Input: part model. Units: mm. Frame: model coordinates. A direction names the side the tool comes from. Coordinates: 2 decimals unless noted, no trailing zeros. Loops run counter-clockwise (first coordinate to the right, second up) from the corner with the lowest first, then second, coordinate; pieces in that order, holes last. Notation, with made-up numbers: (30.5, 40.5) -> (60.5, 40.5) arc R10 cw to (60.5, 50.5) -> close; hole circle Ø5 at (-35, 66). An arc over 180 degrees is marked (long way). Answer as a JSON object with one key per item and string values.
from build123d import *

# Parameters (mm, degrees)
BOSS_EXTRUDE1_DEPTH                 = 31.75
SKETCH3_W                           = 25.4
SKETCH3_H                           = 25.4
CUT_EXTRUDE1_DEPTH                  = 25.4
CUT_EXTRUDE2_DEPTH                  = 30.48
SKETCH5_W                           = 2.54
SKETCH5_H                           = 2.54
BOSS_EXTRUDE2_DEPTH                 = 2.032
SKETCH7_W                           = 2.54
SKETCH7_H                           = 2.54
BOSS_EXTRUDE3_DEPTH                 = 2.032
FILLET1_R                           = 2.54
FILLET2_R                           = 2.54
TAP_DRILL_FOR_6_32_TAP1_D           = 2.7051
TAP_DRILL_FOR_6_32_TAP1_CSINK_D     = 3.9751
TAP_DRILL_FOR_6_32_TAP1_CSINK_ANGLE = 90
TAP_DRILL_FOR_6_32_TAP2_D           = 2.7051
TAP_DRILL_FOR_6_32_TAP2_CSINK_D     = 3.9751
TAP_DRILL_FOR_6_32_TAP2_CSINK_ANGLE = 90


with BuildPart() as part:
    # Sketch1 → Boss-Extrude1 (new, symmetric)
    with BuildSketch(Plane(origin=(0, 0, 0), x_dir=(1, 0, 0), z_dir=(0, 1, 0))):
        with BuildLine():
            Line((-4.43094419, 12.953042159), (-15.24, 12.953042159))
            Line((-15.24, 12.953042159), (-15.24, -16.51))
            Line((-15.24, -16.51), (15.24, -16.51))
            Line((15.24, -16.51), (15.24, 12.953042159))
            Line((15.24, 12.953042159), (4.43094419, 12.953042159))
            ThreePointArc((4.43094419, 12.953042159), (0, 12.82766418), (-4.43094419, 12.953042159))
        make_face()
        with BuildLine():
            Line((-15.24, 14.323960084), (-15.24, 12.953042159))
            Line((-15.24, 12.953042159), (-4.43094419, 12.953042159))
            ThreePointArc((-4.43094419, 12.953042159), (-9.859328847, 13.450401628), (-15.24, 14.323960084))
        make_face()
        with BuildLine():
            ThreePointArc((15.24, 14.323960084), (9.859328847, 13.450401628), (4.43094419, 12.953042159))
            Line((4.43094419, 12.953042159), (15.24, 12.953042159))
            Line((15.24, 12.953042159), (15.24, 14.323960084))
        make_face()
    extrude(amount=BOSS_EXTRUDE1_DEPTH, both=True)

    # Sketch3 → Cut-Extrude1 (cut)
    with BuildSketch(Plane.XY.offset(16.51)):
        with Locations((0, -16.51)):
            Rectangle(SKETCH3_W, SKETCH3_H)
    extrude(amount=-CUT_EXTRUDE1_DEPTH, mode=Mode.SUBTRACT)

    # Sketch4 → Cut-Extrude2 (cut)
    with BuildSketch(Plane(origin=(15.24, 0, 0), x_dir=(0, 0, -1), z_dir=(1, 0, 0))):
        Polygon((-16.51, 31.75), (14.323960084, 31.75), (-16.51, 0), align=None)
    extrude(amount=-CUT_EXTRUDE2_DEPTH, mode=Mode.SUBTRACT)

    # Sketch5 → Boss-Extrude2 (add)
    with BuildSketch(Plane(origin=(15.24, 0, 0), x_dir=(0, 0, -1), z_dir=(1, 0, 0))):
        with Locations((-13.616039916, -25.4)):
            Rectangle(SKETCH5_W, SKETCH5_H)
        with Locations((-13.616039916, -15.24)):
            Rectangle(SKETCH5_W, SKETCH5_H)
    extrude(amount=BOSS_EXTRUDE2_DEPTH)

    # Sketch7 → Boss-Extrude3 (add)
    with BuildSketch(Plane.ZY.offset(15.24)):
        with Locations((13.616039916, -25.4)):
            Rectangle(SKETCH7_W, SKETCH7_H)
        with Locations((13.616039916, -15.24)):
            Rectangle(SKETCH7_W, SKETCH7_H)
    extrude(amount=BOSS_EXTRUDE3_DEPTH)

    # Sketch21 → #1 (0.228) Diameter Hole3 (revolve, cut)
    with BuildSketch(Plane(origin=(0, -3.81, 3.81), x_dir=(0, 0, -1), z_dir=(1, 0, 0))):
        Polygon((0, 0), (0, 35.56), (2.8956, 35.56), (2.8956, 0.12065), (3.01625, 0), align=None)
    revolve(axis=Axis((0, -10.16, 3.81), (0, 1, 0)), mode=Mode.SUBTRACT)

    # Fillet1
    fillet1_edges = [part.edges().sort_by_distance(p)[0] for p in [
        (0, 0, 16.51),
    ]]
    fillet(fillet1_edges, radius=FILLET1_R)

    # Fillet2
    fillet2_edges = [part.edges().sort_by_distance(p)[0] for p in [
        (0, -31.75, 16.51),
    ]]
    fillet(fillet2_edges, radius=FILLET2_R - 0.0001)  # a hair under: the kernel refuses the full size

    # Tap Drill for #6-32 Tap1 (through all)
    with Locations(Plane.XY.offset(-8.89)):
        with Locations((-8.688147052, -16.814161917)):
            CounterSinkHole(TAP_DRILL_FOR_6_32_TAP1_D / 2, TAP_DRILL_FOR_6_32_TAP1_CSINK_D / 2, counter_sink_angle=TAP_DRILL_FOR_6_32_TAP1_CSINK_ANGLE)

    # Tap Drill for #6-32 Tap2 (through all)
    with Locations(Plane.XY.offset(-8.89)):
        with Locations((8.657032922, -16.667582931)):
            CounterSinkHole(TAP_DRILL_FOR_6_32_TAP2_D / 2, TAP_DRILL_FOR_6_32_TAP2_CSINK_D / 2, counter_sink_angle=TAP_DRILL_FOR_6_32_TAP2_CSINK_ANGLE)


solid = part.part
1. Section query C-C (y = 9.5). Return loops of the section in (x, z).
Reply:
{"outline": "(-15.24, -14.32) arc R78.36 cw to (15.24, -14.32) -> (15.24, 7.28) -> (-15.24, 7.28) -> close; hole circle Ø5.79 at (0, 3.81)"}
2. Section query A-A (z = -4.5). Return loops of the section in (x, y).
Reply:
{"outline": "(-15.24, -31.75) -> (15.24, -31.75) -> (15.24, 21.63) -> (-15.24, 21.63) -> close; hole (-12.7, -29.21) -> (12.7, -29.21) -> (12.7, -3.81) -> (-12.7, -3.81) -> close"}
3. Access query for faces 1 (the face through (-16, -15, 14.886)), 2 (the face through (-16, -24.13, 14)), 3 (the face through (16, -25, 14.886)). Directions: +Z, -Z, +X, -X, +Y, -Y. A direction counts if a zero-diameter tool reaches every point of the face in a straight line with its end or side. Return the directions, or none.
Reply:
{"face 1": "+Z, -X, +Y, -Y", "face 2": "+Z, -Z, -X", "face 3": "+Z, +X, +Y, -Y"}
4. Pin query (flat end, axial travel): P1, Ø1, axis at x = -16.5, y = -15.5, coming from the +Z side; P2, Ø4, axis at x = 12, y = 9.5, coming from the +Z side; P3, Ø2, axis at x = -16.5, z = 14, coming from the -Y side; P4, Ø1.5, axis at y = 22, z = -3, coming from the +X side. Return the tip coordinate at first contact, or that it passes through.
Reply:
{"P1": "stops at z = 14.89", "P2": "stops at z = 9.23", "P3": "stops at y = -26.67", "P4": "passes through"}
5. Mould query, pull axis X, two halves, no side actions, for faces 4 (the face through (-12.7, -17, 4)), 5 (the face through (0, -29.21, 4)), 6 (the face through (16, -15, 14.886)), 7 (the face through (17.272, -15, 14)). Classes: pulls with the +X half, pulls with the -X half, needs draft (parallel to the pull), parting line crosses it, or undercut.
Reply:
{"face 4": "undercut", "face 5": "undercut", "face 6": "needs draft", "face 7": "pulls with the +X half"}
6. Line query: line 1 along X through (y, z) = (-14, 5); line 2 along Y through (x, z) = (0, -6.5); line 3 along X through (y, z) = (0.5, -5). Output: solid intervals per line, ascending.
Reply:
{"line 1": "x = -15.24 to -12.7, 12.7 to 15.24", "line 2": "y = -31.75 to -29.21, -3.81 to 23.69", "line 3": "x = -15.24 to 15.24"}
7. Section query D-D (z = 3.81). Return loops of the section in (x, y), plus the area to 3 significant figures.
Reply:
{"outline": "(-15.24, -31.75) -> (15.24, -31.75) -> (15.24, 13.08) -> (2.9, 13.08) -> (2.9, -3.69) -> (3.02, -3.81) -> (12.7, -3.81) -> (12.7, -29.21) -> (-12.7, -29.21) -> (-12.7, -3.81) -> (-3.02, -3.81) -> (-2.9, -3.69) -> (-2.9, 13.08) -> (-15.24, 13.08) -> close", "area": "623 mm2"}
